```python
from build123d import *

# Parameters (mm, degrees)
SKETCH_W     = 41
SKETCH_H     = 10.25
PAD_DEPTH    = 2
PAD001_DEPTH = 25
SKETCH003_R  = 1.65
POCKET_DEPTH = 102.301798
CHAMFER_SIZE = 4


with BuildPart() as part:
    # Sketch → Pad (new body)
    with BuildSketch(Plane.XY):
        with Locations((0, 5.125)):
            Rectangle(SKETCH_W, SKETCH_H)
    extrude(amount=PAD_DEPTH)

    # Sketch002 (on Face6 of Pad) → Pad001 (join)
    with BuildSketch(Plane.XY.offset(2)):
        Polygon((16.5, 4.5), (20.5, 4.5), (20.5, 0), (16.5, 0), (16.5, 1.45), (19.5, 1.45), (19.5, 3.05), (16.5, 3.05), align=None)
    pad001 = extrude(amount=PAD001_DEPTH)

    # Sketch003 (on Face5 of Pad001) → Pocket (cut, through all)
    with BuildSketch(Plane.XY.offset(2)):
        with Locations((10, 7.375)):
            Circle(SKETCH003_R)
    pocket = extrude(amount=-POCKET_DEPTH, mode=Mode.SUBTRACT)

    # Mirrored: Pocket, Pad001 across Sketch003 V_Axis
    add(pocket.mirror(Plane(origin=(0, 0, 2), x_dir=(0, 0, 1), z_dir=(1, 0, 0))), mode=Mode.SUBTRACT)
    add(pad001.mirror(Plane(origin=(0, 0, 2), x_dir=(0, 0, 1), z_dir=(1, 0, 0))))

    # Chamfer
    chamfer_edges = [part.edges().sort_by_distance(p)[0] for p in [
        (18.5, 4.5, 2),
        (-18.5, 4.5, 2),
    ]]
    chamfer(chamfer_edges, length=CHAMFER_SIZE)


solid = part.part
```
CAD build for the part. Positions are in the model's coordinates, mm. A direction names the side the tool comes from. Coordinates: 2 decimals unless noted, no trailing zeros. Order: outer loops, then holes, each group sorted by start corner. A loop starts at its lowest first (then second) coordinate and runs counter-clockwise, first axis right, second up. Notation, with made-up numbers: (-2.75, 41.25) - (37.25, 41.25) arc R16 ccw to (37.25, 47.25) - close; hole circle Ø5 at (26, 5). An arc over 180 degrees is marked (long way). Answer in a Markdown table with one row per item.
1. 3-axis set-ups, long thin cutter, end or side, ignore diameter. For faces 5 (the face through (18, 3.05, 14)), 6 (the face through (-19, 1, 27)), 7 (the face through (-16.5, 4, 13)), 8 (the face through (11.524, 6.743, 1.014)), 9 (the face through (-18, 4.5, 16)): which of +Z, -Z, +X, -X, +Y, -Y reach the whole face in a straight line?
Answer:
| item | result |
|---|---|
| face 5 | +Z |
| face 6 | +Z, +X, -X, +Y, -Y |
| face 7 | +Z, +Y, -Y |
| face 8 | +Z, -Z |
| face 9 | +Z, +X, -X, +Y |
2. Slice it at B-B, the plane x = -10. List the corners of the cut face in (y, z) (3 decimals), then the cut area to 3 significant figures.
Answer:
| item | result |
|---|---|
| outline | (0, 0) - (5.725, 0) - (5.725, 2) - (0, 2) - close; (9.025, 0) - (10.25, 0) - (10.25, 2) - (9.025, 2) - close |
| area | 13.9 mm² |
3. Slice it at A-A, the plane z = 3. List the corners of the cut face in (x, y).
Answer:
| item | result |
|---|---|
| outline | (-20.5, 0) - (-16.5, 0) - (-16.5, 1.45) - (-19.5, 1.45) - (-19.5, 3.05) - (-16.5, 3.05) - (-16.5, 7.5) - (-20.5, 7.5) - close; (16.5, 0) - (20.5, 0) - (20.5, 7.5) - (16.5, 7.5) - (16.5, 3.05) - (19.5, 3.05) - (19.5, 1.45) - (16.5, 1.45) - close |
4. Flat gauge pins, fed straight in: P1, Ø1, axis at y = 6, z = 20.5, coming from the +X side; P2, Ø0.9, axis at x = 17.5, z = 16.5, coming from the +Y side; P3, Ø5, axis at x = -4.5, y = 3.5, coming from the +Z side. Where does each tip first touch, or does it go through?
Answer:
| item | result |
|---|---|
| P1 | through |
| P2 | y = 4.5 |
| P3 | z = 2 |
5. Slice it at C-C, the plane y = 0.5. List the corners of the cut face in (x, z).
Answer:
| item | result |
|---|---|
| outline | (-20.5, 0) - (20.5, 0) - (20.5, 27) - (16.5, 27) - (16.5, 2) - (-16.5, 2) - (-16.5, 27) - (-20.5, 27) - close |
6. Drill centre lines: L1, parallel to Y at x = 10, z = 0.55 (3 decimals); L2, parallel to X at y = 1.25, z = 23.25; L3, parallel to Y at x = -18.5, z = 20.5. Where is each one in solid material? Low to high. Write a range as from..to.
Answer:
| item | result |
|---|---|
| L1 | 0..5.725, 9.025..10.25 |
| L2 | -20.5..-16.5, 16.5..20.5 |
| L3 | 0..1.45, 3.05..4.5 |
7. Slice it at D-D, the plane z = 9.5. List the corners of the cut face in (x, y).
Answer:
| item | result |
|---|---|
| outline | (-20.5, 0) - (-16.5, 0) - (-16.5, 1.45) - (-19.5, 1.45) - (-19.5, 3.05) - (-16.5, 3.05) - (-16.5, 4.5) - (-20.5, 4.5) - close; (16.5, 0) - (20.5, 0) - (20.5, 4.5) - (16.5, 4.5) - (16.5, 3.05) - (19.5, 3.05) - (19.5, 1.45) - (16.5, 1.45) - close |
8. Pull direction X, two halves, no side cores. Call faces 1 (the face through (0, 10.25, 1)), 2 (the face through (20.5, 3, 10)), 3 (the face through (-16.5, 1, 14)), 4 (the face through (16.5, 4, 13)): +X half, -X half, draft (parallel to the pull), parting line (faces both ways), or undercut.
Answer:
| item | result |
|---|---|
| face 1 | draft |
| face 2 | +X half |
| face 3 | undercut |
| face 4 | undercut |
